Work out the finished part from the listing and answer in its coordinate system (mm). Give positions to 0.01 mm unless a question says otherwise; leave off trailing zeros. Write each loop counter-clockwise with the first axis right and the second up, starting at its lowest first coordinate (ties: lowest second). Pieces come first, ordered by that corner, then holes. Notation, with made-up numbers: (-38, -0.75) -> (-23, -0.75) arc R15 cw to (-23, 20.25) -> close; hole circle Ø7 at (49, -27). An arc over 180 degrees is marked (long way). Use a Markdown table: item, result. Add a question column.
Q1. Section A-A, the plane y = 0 is taken. Give the vertices of the cut face in (x, z), plus the area to 3 significant figures.
Q2. For a pull along X with two mould halves and no side action, classify faces 1 (the face through (-9.764, 74.362, 0.493)), 2 (the face through (16, 34, 1)), 3 (the face through (-8.02, -36.12, 0.49)) as pulls with the +X half, pulls with the -X half, needs draft (parallel to the pull), parting line crosses it, or undercut.
Q3. Consider line 1 (Y direction, x = 0, z = 0.55); line 2 (Y direction, x = -28.5, z = 0.1); line 3 (Y direction, x = 39, z = 0.1). Determine where each line is inside the solid, lowest interval first.
Q4. Section C-C, the plane z = 0.35 is taken. State how many separate pieces and enclosed holes the cut face has, plus the area to 3 significant figures.
Q5. Section B-B, the plane x = -14.5 is taken. Give the vertices of the cut face in (y, z), plus the area to 3 significant figures.
Q6. Each of these flat-tipped pins is pushed along its axis until it touches: pin 1 Ø0.5 at (y, z) = (-68, 0.5) entering from +X; pin 2 Ø0.5 at (y, z) = (-53, 0.5) entering from -X; pin 3 Ø0.5 at (x, z) = (-0.5, 0.5) entering from +Y. Where does it stop, or does it pass through?
Q7. Section D-D, the plane y = 65 is taken. Give the vertices of the cut face in (x, z).
from build123d import *

# Parameters (mm, degrees)
SKETCH1_R           = 75
SKETCH1_R_2         = 37
SKETCH1_R_3         = 1.5
SKETCH1_W           = 3
SKETCH1_H           = 5
BOSS_EXTRUDE1_DEPTH = 1


with BuildPart() as part:
    # Sketch1 → Boss-Extrude1 (new body)
    with BuildSketch(Plane.XY):
        Circle(SKETCH1_R)
        Circle(SKETCH1_R_2, mode=Mode.SUBTRACT)
        with Locations((0, -60)):
            Circle(SKETCH1_R_3, mode=Mode.SUBTRACT)
        with Locations((54.378467222, 25.357095704)):
            Circle(SKETCH1_R_3, mode=Mode.SUBTRACT)
        with Locations((-54.378467222, 25.357095704)):
            Circle(SKETCH1_R_3, mode=Mode.SUBTRACT)
        with Locations((0, -52.5)):
            Rectangle(SKETCH1_W, SKETCH1_H, mode=Mode.SUBTRACT)
        with Locations((0, -67.5)):
            Rectangle(SKETCH1_W, SKETCH1_H, mode=Mode.SUBTRACT)
        Polygon((49.213000894, 24.603466076), (44.681461959, 22.490374768), (45.949316744, 19.771451406), (50.48085568, 21.884542715), align=None, mode=Mode.SUBTRACT)
        Polygon((58.276078765, 28.829648694), (62.8076177, 30.942740002), (64.075472485, 28.223816641), (59.54393355, 26.110725333), align=None, mode=Mode.SUBTRACT)
        Polygon((-58.276078765, 28.829648694), (-62.8076177, 30.942740002), (-64.075472485, 28.223816641), (-59.54393355, 26.110725333), align=None, mode=Mode.SUBTRACT)
        Polygon((-49.213000894, 24.603466076), (-44.681461959, 22.490374768), (-45.949316744, 19.771451406), (-50.48085568, 21.884542715), align=None, mode=Mode.SUBTRACT)
    extrude(amount=BOSS_EXTRUDE1_DEPTH)


solid = part.part
Result set:
| question | item | result |
|---|---|---|
| 1 | outline | (-75, 0) -> (-37, 0) -> (-37, 1) -> (-75, 1) -> close; (37, 0) -> (75, 0) -> (75, 1) -> (37, 1) -> close |
| 1 | area | 76.0 mm2 |
| 2 | face 1 | parting line crosses it |
| 2 | face 2 | needs draft |
| 2 | face 3 | undercut |
| 3 | line 1 | y = -75 to -70, -65 to -61.5, -58.5 to -55, -50 to -37, 37 to 75 |
| 3 | line 2 | y = -69.37 to -23.6, 23.6 to 69.37 |
| 3 | line 3 | y = -64.06 to 64.06 |
| 4 | separate pieces | 1 |
| 4 | enclosed holes | 10 |
| 4 | area | 13,300 mm2 |
| 5 | outline | (-73.58, 0) -> (-34.04, 0) -> (-34.04, 1) -> (-73.58, 1) -> close; (34.04, 0) -> (73.58, 0) -> (73.58, 1) -> (34.04, 1) -> close |
| 5 | area | 79.1 mm2 |
| 6 | pin 1 | stops at x = 32.17 |
| 6 | pin 2 | stops at x = -53.31 |
| 6 | pin 3 | stops at y = 75 |
| 7 | outline | (-37.42, 0) -> (37.42, 0) -> (37.42, 1) -> (-37.42, 1) -> close |
